Design review of the part built by this model. Coordinates are the model's own, in mm. Round coordinates to 2 decimals unless told otherwise and drop trailing zeros. Write each loop counter-clockwise with the first axis right and the second up, starting at its lowest first coordinate (ties: lowest second). Pieces come first, ordered by that corner, then holes.
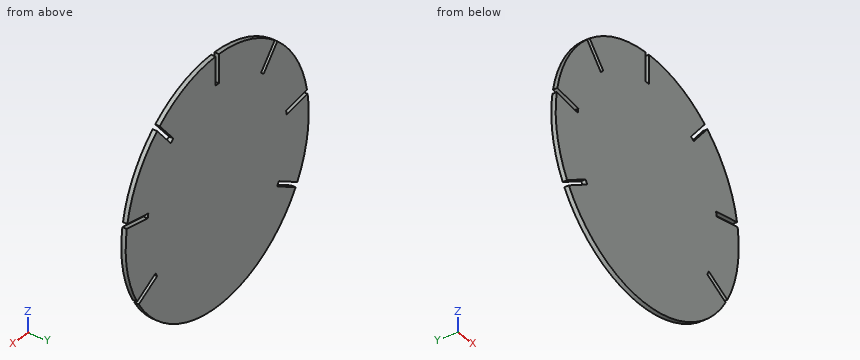
from build123d import *

# Parameters (mm, degrees)
SKETCH1_R           = 185
BOSS_EXTRUDE1_DEPTH = 6.7
SKETCH2_W           = 6.7
SKETCH2_H           = 44
CUT_EXTRUDE3_DEPTH  = 6.7


with BuildPart() as part:
    # Sketch1 → Boss-Extrude1 (new body)
    with BuildSketch(Plane(origin=(0, 0, 0), x_dir=(1, 0, 0), z_dir=(0, 1, 0))):
        with Locations(Location((0, 0, 0), (0, 0, 270))):
            Circle(SKETCH1_R)
    extrude(amount=BOSS_EXTRUDE1_DEPTH)

    # Sketch2 → Cut-Extrude3 (cut)
    with BuildSketch(Plane(origin=(0, 6.7, 0), x_dir=(1, 0, 0), z_dir=(0, 1, 0))):
        Polygon((159.405725104, 95.901185103), (121.300607337, 73.901185103), (124.650607337, 68.098814897), (162.755725104, 90.098814897), align=None)
        Polygon((122.124744286, -140.330927928), (93.84208946, -106.62497243), (88.709591691, -110.931649415), (116.992246517, -144.637604913), align=None)
        Polygon((183.755963455, -28.999455073), (140.424422323, -21.358935256), (139.260979533, -27.957147201), (182.592520665, -35.597667019), align=None)
        with Locations((0, -164)):
            Rectangle(SKETCH2_W, SKETCH2_H)
        Polygon((-116.992246517, -144.637604913), (-88.709591691, -110.931649415), (-93.84208946, -106.62497243), (-122.124744286, -140.330927928), align=None)
        Polygon((-182.592520665, -35.597667019), (-139.260979533, -27.957147201), (-140.424422323, -21.358935256), (-183.755963455, -28.999455073), align=None)
        Polygon((-162.755725104, 90.098814897), (-124.650607337, 68.098814897), (-121.300607337, 73.901185103), (-159.405725104, 95.901185103), align=None)
    extrude(amount=-CUT_EXTRUDE3_DEPTH, mode=Mode.SUBTRACT)


solid = part.part
1) For line 1 along Z through (x, y) = (-142.5, 4.5); line 2 along X through (y, z) = (3, 136.5); line 3 along X through (y, z) = (2.75, 111), list the stretches that pass through material, from the lowest coordinate up.
2) For P1, Ø3.5, axis at x = -1.5, y = 5, coming from the +Z side; P2, Ø4, axis at x = -93, y = 2.5, coming from the -Z side; P3, Ø1.5, axis at x = 120.5, y = 4.5, coming from the -Z side, all flat-tipped, find the tip position at first contact; note any pin that passes through.
3) Add section C-C on z = 60. State the section outline as (x, y) points, and give its area (4 significant figures).
4) Add section B-B on z = -79. State the section outline as (x, y) points, and give its area (3 significant figures).
5) Add section D-D on x = 60.5. State the section outline as (y, z) points, and give its area (3 significant figures).
6) Add section A-A on y = 4.5. State the section outline as (x, z) points.
Computed:
1. line 1: z = -117.98 to -86.14, -78.4 to 21.72, 28.53 to 117.98
1. line 2: x = -124.87 to -118.91, -110.16 to 110.16, 118.91 to 124.87
1. line 3: x = -148 to -97.51, -88.77 to 88.77, 97.51 to 148
2. P1: stops at z = 142
2. P2: stops at z = -161.07
2. P3: stops at z = -141.01
3. outline: (-175, 0) - (175, 0) - (175, 6.7) - (-175, 6.7) - close
3. area: 2,345 mm2
4. outline: (-167.28, 0) - (-143.53, 0) - (-143.53, 6.7) - (-167.28, 6.7) - close; (-130.13, 0) - (130.13, 0) - (130.13, 6.7) - (-130.13, 6.7) - close; (143.53, 0) - (167.28, 0) - (167.28, 6.7) - (143.53, 6.7) - close
4. area: 2,060 mm2
5. outline: (0, -174.83) - (6.7, -174.83) - (6.7, 174.83) - (0, 174.83) - close
5. area: 2,340 mm2
6. outline: (-182.74, 28.82) arc R185 ccw to (-161.86, -89.58) - (-124.65, -68.1) - (-121.3, -73.9) - (-158.51, -95.39) arc R185 ccw to (158.51, -95.39) - (121.3, -73.9) - (124.65, -68.1) - (161.86, -89.58) arc R185 ccw to (182.74, 28.82) - (140.42, 21.36) - (139.26, 27.96) - (181.58, 35.42) arc R185 ccw to (121.46, 139.54) - (93.84, 106.62) - (88.71, 110.93) - (116.33, 143.85) arc R185 ccw to (3.35, 184.97) - (3.35, 142) - (-3.35, 142) - (-3.35, 184.97) arc R185 ccw to (-116.33, 143.85) - (-88.71, 110.93) - (-93.84, 106.62) - (-121.46, 139.54) arc R185 ccw to (-181.58, 35.42) - (-139.26, 27.96) - (-140.42, 21.36) - close
